Model file for the job. Use its own axes, mm. A direction names the side the tool comes from. Round coordinates to 2 decimals unless told otherwise and drop trailing zeros. Loops run counter-clockwise (first coordinate to the right, second up) from the corner with the lowest first, then second, coordinate; pieces in that order, holes last. Notation, with made-up numbers: M -8.5,-36.5 L 43.5,-36.5 A11 ccw 43.5,-28.5 Z; hole C 79.25,10 d2. An arc over 180 degrees is marked long. Use a Markdown table: item, result. Add a question column.
Q1. Cut at A-A (z = -293). Give the cut face in (x, y), plus the area to 3 significant figures.
Q2. Probe line 1 (X direction, y = 13, z = -50.5); line 2 (Z direction, x = -74, y = 12); line 3 (X direction, y = -19, z = -114.5). List the from-to ranges inside material, lowest first. Write a range as from..to.
Q3. Pin check, flat tip, straight feed: pin 1 (8 mm diameter, centred on x = -319.5, z = 337, fed in from +Y). Stop position of the tip, or through.
Q4. Tool access for faces 3 (the face through (2, -9, -319.5)), 4 (the face through (-212, 0, -114)), 5 (the face through (-216, -9, 31.5)): list every direction of +Z, -Z, +X, -X, +Y, -Y with a clear straight run to the whole face (end or side of a thin tool).
Q5. Cut at B-B (x = 3.5). Give the cut face in (y, z).
Q6. Cut at D-D (z = 91). Give the cut face in (x, y), plus the area to 3 significant figures.
Q7. Cut at C-C (y = 6.5). Give the cut face in (x, z).
Q8. Mould opens along X. For faces 1 (the face through (-2, 18, 2)), 2 (the face through (-214, 9, 126.5)) say: +X half, -X half, draft (parallel to the pull), parting line (faces both ways), or undercut.
from build123d import *

# Parameters (mm, degrees)
F0_W     = 55
F0_H     = 178
F0_W_2   = 58
F0_W_3   = 59
F0_W_4   = 70
F0_H_2   = 18
F1_DEPTH = 18
F0_W_5   = 780
F0_W_6   = 800
F0_H_3   = 885
F2_DEPTH = 25
F0_W_7   = 357
F0_H_4   = 70
F0_W_8   = 353
F0_H_5   = 351
F0_H_6   = 95
F0_H_7   = 77
F3_DEPTH = 18


# Not quite as in the source:
# - a feature names something its author has since deleted; it is built from what else it names


with BuildPart() as f1:
    # F0 (on Front) → F1 (new body)
    with BuildSketch(Plane.XZ):
        Polygon((-299, 49.5), (-390, 49.5), (-390, 40.5200137198), (-390, 31.5), (-299, 31.5), (-299, -38.5), (-299, -56.5), (-299, -234.5), (-299, -252.5), (-299, -319.5), (-390, -319.5), (-390, -337.5), (-299, -337.5), (-281, -337.5), (-150, -337.5), (-132, -337.5), (-33, -337.5), (-33, -319.5), (-132, -319.5), (-132, -252.5), (-132, -234.5), (-132, -56.5), (-132, -38.5), (-132, 31.5), (-33, 31.5), (-33, 49.5), (-132, 49.5), (-150, 49.5), (-281, 49.5), align=None)
        Polygon((-226, -252.5), (-208, -252.5), (-150, -252.5), (-150, -319.5), (-281, -319.5), (-281, -252.5), align=None, mode=Mode.SUBTRACT)
        with Locations((-253.5, -145.5)):
            Rectangle(F0_W, F0_H, mode=Mode.SUBTRACT)
        Polygon((-281, 31.5), (-150, 31.5), (-150, -38.5), (-208, -38.5), (-226, -38.5), (-281, -38.5), align=None, mode=Mode.SUBTRACT)
        with Locations((-179, -145.5)):
            Rectangle(F0_W_2, F0_H, mode=Mode.SUBTRACT)
        Polygon((390, 40.5200137198), (390, 49.5), (301, 49.5), (283, 49.5), (151, 49.5), (133, 49.5), (37, 49.5), (37, 31.5), (133, 31.5), (133, -38.5), (133, -56.5), (133, -234.5), (133, -252.5), (133, -319.5), (37, -319.5), (37, -337.5), (133, -337.5), (151, -337.5), (283, -337.5), (301, -337.5), (390, -337.5), (390, -319.5), (301, -319.5), (301, -252.5), (301, -234.5), (301, -56.5), (301, -38.5), (301, 31.5), (390, 31.5), align=None)
        Polygon((206, -252.5), (224, -252.5), (283, -252.5), (283, -319.5), (151, -319.5), (151, -252.5), align=None, mode=Mode.SUBTRACT)
        with Locations((178.5, -145.5)):
            Rectangle(F0_W, F0_H, mode=Mode.SUBTRACT)
        with Locations((253.5, -145.5)):
            Rectangle(F0_W_3, F0_H, mode=Mode.SUBTRACT)
        Polygon((151, 31.5), (283, 31.5), (283, -38.5), (224, -38.5), (206, -38.5), (151, -38.5), align=None, mode=Mode.SUBTRACT)
        with Locations((2, 40.5)):
            Rectangle(F0_W_4, F0_H_2)
        with Locations((2, -328.5)):
            Rectangle(F0_W_4, F0_H_2)
    extrude(amount=F1_DEPTH)



with BuildPart() as f1b:
    # F0 (on Front) → F1, piece 2 (new body)
    with BuildSketch(Plane.XZ):
        with Locations((0, 327.5)):
            Rectangle(F0_W_5, F0_H_2)
    extrude(amount=F1_DEPTH)


with BuildPart() as f1_1:
    add(f1.part)

    add(f1b.part)  # F2 merges F1b
    # F0 (on Front) → F2 (join)
    with BuildSketch(Plane.XZ):
        Rectangle(F0_W_6, F0_H_3)
        Polygon((-390, 432.5), (390, 432.5), (390, 336.5), (390, 318.5), (390, 196.5), (390, 126.5), (390, 49.5), (390, 40.5200137198), (390, 31.5), (390, -38.5), (390, -56.5), (390, -234.5), (390, -252.5), (390, -319.5), (390, -337.5), (390, -432.5), (37, -432.5), (-33, -432.5), (-390, -432.5), (-390, -337.5), (-390, -319.5), (-390, -252.5), (-390, -234.5), (-390, -140.5), (-390, -56.5), (-390, -38.5), (-390, 31.5), (-390, 40.5200137198), (-390, 49.5), (-390, 126.5), (-390, 196.5), (-390, 318.5), (-390, 336.5), align=None, mode=Mode.SUBTRACT)
    extrude(amount=F2_DEPTH)

    # F0 (on Front) → F3 (join)
    with BuildSketch(Plane.XZ):
        Rectangle(F0_W_6, F0_H_3)
        Polygon((-390, 432.5), (390, 432.5), (390, 336.5), (390, 318.5), (390, 196.5), (390, 126.5), (390, 49.5), (390, 40.5200137198), (390, 31.5), (390, -38.5), (390, -56.5), (390, -234.5), (390, -252.5), (390, -319.5), (390, -337.5), (390, -432.5), (37, -432.5), (-33, -432.5), (-390, -432.5), (-390, -337.5), (-390, -319.5), (-390, -252.5), (-390, -234.5), (-390, -140.5), (-390, -56.5), (-390, -38.5), (-390, 31.5), (-390, 40.5200137198), (-390, 49.5), (-390, 126.5), (-390, 196.5), (-390, 318.5), (-390, 336.5), align=None, mode=Mode.SUBTRACT)
        with Locations((-211.5, 161.5)):
            Rectangle(F0_W_7, F0_H_4)
        with Locations((213.5, 161.5)):
            Rectangle(F0_W_8, F0_H_4)
        with Locations((2, -144)):
            Rectangle(F0_W_4, F0_H_5)
        with Locations((2, -385)):
            Rectangle(F0_W_4, F0_H_6)
        with Locations((2, 88)):
            Rectangle(F0_W_4, F0_H_7)
        with Locations((2, 161.5)):
            Rectangle(F0_W_4, F0_H_4)
        with Locations((2, 40.5)):
            Rectangle(F0_W_4, F0_H_2)
        with Locations((2, -328.5)):
            Rectangle(F0_W_4, F0_H_2)
    extrude(amount=-F3_DEPTH)


solid = f1_1.part
Checked values:
| question | item | result |
|---|---|---|
| 1 | outline | M -400,-25 L -390,-25 L -390,18 L -400,18 Z; M -299,-18 L -281,-18 L -281,0 L -299,0 Z; M -150,-18 L -132,-18 L -132,0 L -150,0 Z; M -33,0 L 37,0 L 37,18 L -33,18 Z; M 133,-18 L 151,-18 L 151,0 L 133,0 Z; M 283,-18 L 301,-18 L 301,0 L 283,0 Z; M 390,-25 L 400,-25 L 400,18 L 390,18 Z |
| 1 | area | 3,420 mm^2 |
| 2 | line 1 | x = -400..-390, -33..37, 390..400 |
| 2 | line 2 | z = -442.5..-432.5, 126.5..196.5, 432.5..442.5 |
| 2 | line 3 | x = -400..-390, 390..400 |
| 3 | pin 1 | stops at y = 0 |
| 4 | face 3 | -Y |
| 4 | face 4 | +Y |
| 4 | face 5 | +Y, -Y |
| 5 | outline | M -25,-442.5 L 18,-442.5 L 18,196.5 L 0,196.5 L 0,49.5 L -18,49.5 L -18,31.5 L 0,31.5 L 0,-319.5 L -18,-319.5 L -18,-337.5 L 0,-337.5 L 0,-432.5 L -25,-432.5 Z; M -25,432.5 L 18,432.5 L 18,442.5 L -25,442.5 Z; M -18,318.5 L 0,318.5 L 0,336.5 L -18,336.5 Z |
| 6 | outline | M -400,-25 L -390,-25 L -390,18 L -400,18 Z; M -33,0 L 37,0 L 37,18 L -33,18 Z; M 390,-25 L 400,-25 L 400,18 L 390,18 Z |
| 6 | area | 2,120 mm^2 |
| 7 | outline | M -400,-442.5 L 400,-442.5 L 400,442.5 L -400,442.5 Z; hole M -390,-432.5 L -33,-432.5 L -33,126.5 L -390,126.5 Z; hole M -390,196.5 L 390,196.5 L 390,432.5 L -390,432.5 Z; hole M 37,-432.5 L 390,-432.5 L 390,126.5 L 37,126.5 Z |
| 8 | face 1 | draft |
| 8 | face 2 | undercut |
